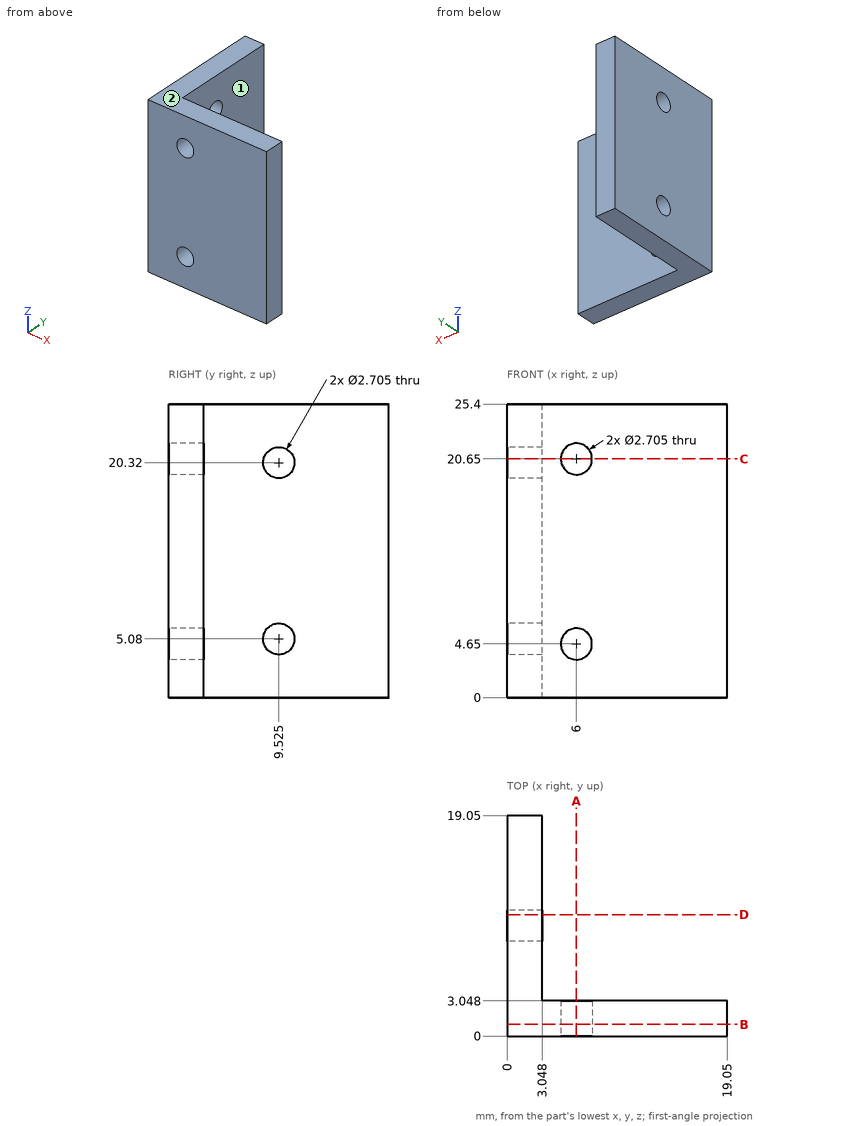
The figure shows three views and two pictorial views of one solid part (mm, origin at its lowest corner). Answer the questions. A direction names the side the tool comes from. Give positions to 0.01 mm unless a question says otherwise; leave off trailing zeros. Write each loop counter-clockwise with the first axis right and the second up, starting at its lowest first coordinate (ties: lowest second). Pieces come first, ordered by that corner, then holes. Notation, with made-up numbers: (22.25, 62) - (79.25, 62) arc R21 ccw to (79.25, 74) - close; hole circle Ø4 at (-26.75, 23.25). An arc over 180 degrees is marked (long way). Return JSON: item names as keys, results as strings.
Q1. A cutting plane is placed at C-C, the plane z = 20.65. Determine the outline of the cut face in (x, y).
Reply:
{"outline": "(0, 0) - (4.65, 0) - (4.65, 3.05) - (3.05, 3.05) - (3.05, 8.21) - (0, 8.21) - close; (0, 10.84) - (3.05, 10.84) - (3.05, 19.05) - (0, 19.05) - close; (7.35, 0) - (19.05, 0) - (19.05, 3.05) - (7.35, 3.05) - close"}
Q2. A cutting plane is placed at A-A, the plane x = 6. Determine the outline of the cut face in (y, z), and give its area (3 significant figures).
Reply:
{"outline": "(0, 0) - (3.05, 0) - (3.05, 3.3) - (0, 3.3) - close; (0, 6) - (3.05, 6) - (3.05, 19.3) - (0, 19.3) - close; (0, 22) - (3.05, 22) - (3.05, 25.4) - (0, 25.4) - close", "area": "60.9 mm²"}
Q3. A cutting plane is placed at D-D, the plane y = 10.5. Determine the outline of the cut face in (x, z).
Reply:
{"outline": "(0, 0) - (3.05, 0) - (3.05, 4.14) - (0, 4.14) - close; (0, 6.02) - (3.05, 6.02) - (3.05, 19.38) - (0, 19.38) - close; (0, 21.26) - (3.05, 21.26) - (3.05, 25.4) - (0, 25.4) - close"}
Q4. Consider line 1 along Z through (x, y) = (6, 0.9); line 2 along Y through (x, z) = (2.35, 5.08); line 3 along Z through (x, y) = (2, 10.25). Determine where each line is inside the solid, lowest interval first. Write a range as [from, to].
Reply:
{"line 1": "[0, 3.3], [6, 19.3], [22, 25.4]", "line 2": "[0, 8.17], [10.88, 19.05]", "line 3": "[0, 3.94], [6.22, 19.18], [21.46, 25.4]"}
Q5. A cutting plane is placed at B-B, the plane y = 1. Count the separate pieces of the cut face and the enclosed holes in it, and give its area (3 significant figures).
Reply:
{"separate pieces": "1", "enclosed holes": "2", "area": "472 mm²"}
Q6. For the marked faces 1 and 2, determine the directions among +Z, -Z, +X, -X, +Y, -Y from which every point of the face is accessible in a straight line to the end or side of a thin tool.
Reply:
{"face 1": "+Z, -Z, +X, +Y", "face 2": "+Z, +X, -X, +Y, -Y"}
Q7. Given P1, Ø1.6, axis at x = 6, z = 4.65, coming from the -Y side; P2, Ø3, axis at x = 5, z = 17.5, coming from the +Y side; P3, Ø3, axis at y = 9.525, z = 5.08, coming from the +X side, each flat-ended and moving along its own axis, determine where each tip first touches the part or whether it passes through.
Reply:
{"P1": "through", "P2": "y = 3.05", "P3": "x = 3.05"}
